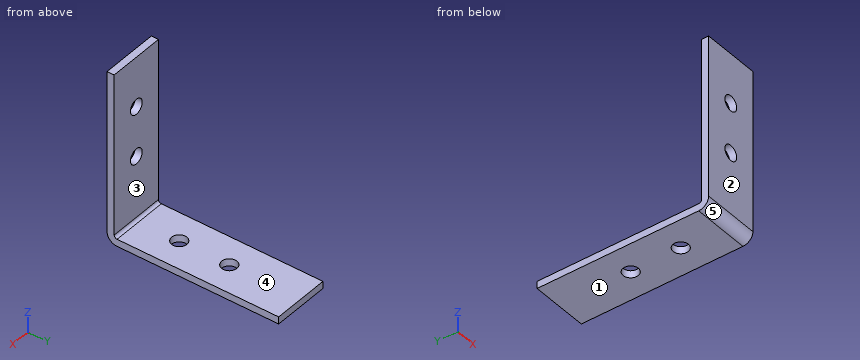
Autodesk Inventor part; units mm, degrees
ref_plane "YZ Plane" through (0, 0, 0) normal (1, 0, 0) x (0, 1, 0)
ref_plane "XZ Plane" through (0, 0, 0) normal (0, 1, 0) x (-1, 0, 0)
ref_plane "XY Plane" through (0, 0, 0) normal (0, 0, 1) x (1, 0, 0)
sketch "Sketch1" plane through (0, 0, 0) normal (0, 0, 1) x (1, 0, 0)
  line L0 (0, 0) -> (147.699314, 0)
  line L1 (147.699314, -25.4) -> (0, -25.4)
  line L2 (0, 0) -> (73.849657, 0)
  line L3 (73.849657, 0) -> (73.849657, -3.175)
  line L4 (73.849657, -3.175) -> (72.249457, -3.175)
  line L5 (72.249457, -3.175) -> (72.249457, -9.525)
  line L6 (72.249457, -9.525) -> (75.424457, -9.525)
  line L7 (75.424457, -9.525) -> (75.424457, -3.175)
  line L8 (75.424457, -3.175) -> (73.849657, -3.175)
  line L9 (73.849657, -25.4) -> (73.849657, -22.225)
  line L10 (73.849657, -22.225) -> (72.249457, -22.225)
  line L11 (72.249457, -22.225) -> (72.249457, -15.875)
  line L12 (72.249457, -15.875) -> (75.424457, -15.875)
  line L13 (75.424457, -15.875) -> (75.424457, -22.225)
  line L14 (75.424457, -22.225) -> (73.849657, -22.225)
  dimension "d8" = 6.7564
sketch "Sketch3" plane through (0, 3.175, 76.2) normal (0, 1, 0) x (1, 0, 0)
  line L0 (0, 0) -> (25.4, 0)
  circle A0 centre (12.7, 44.45) radius 3.3782
  circle A1 centre (12.7, 22.225) radius 3.3782
  line L1 (0, 76.2) -> (0, 73.025)
  dimension "d21" = 6.7564
  dimension "d22" = 6.7564
  dimension "d23" = 12.7
  dimension "d24" = 22.225
  dimension "d25" = 22.225
sketch "Sketch1 outline for Plate1" plane through (0, 0, 0) normal (0, 0, 1) x (1, 0, 0)
  line L0 (0, 0) -> (0, 76.2)
  line L1 (25.4, 0) -> (0, 0)
  line L2 (0, 76.2) -> (25.4, 76.2)
  line L3 (25.4, 76.2) -> (25.4, 0)
  circle A0 centre (12.7, 22.225) radius 3.3782
  circle A1 centre (12.7, 44.45) radius 3.3782
extrude "Plate1" add sketch "Sketch1 outline for Plate1" along normal blind 3.175
sketch "Sketch2" plane through (25.4, 3.175, 0) normal (0, -1, 0) x (1, 0, 0)
  line L0 (-25.4, 0) -> (0, 0)
  line L1 (0, 0) -> (0, 76.2)
  line L2 (0, 76.2) -> (-25.4, 76.2)
  line L3 (-25.4, 76.2) -> (-25.4, 0)
edge flange "Flange1" height 76.2 angle 90 thickness 3.175 bend radius 1.27 thickness toward (0, -1, 0) relief tear relief width 3.175 relief depth 1.5875 edges at (12.7, 0, 3.175) wall of the first edge with corners at (0, 3.175, 0) (25.4, 3.175, 0) (25.4, 3.175, 76.2) (0, 3.175, 76.2)
bend "Bend1"
corner "Corner1"
extrude "Cut1" cut sketch "Sketch3" against normal blind 3.175
equation "\"d11\" = BendReliefWidth"
equation "\"d12\" = BendReliefDepth"
equation "\"d13\" = MinimumRemnant"
equation "\"d14\" = BendRadius"
equation "\"d18\" = CornerReliefSize"
equation "\"d19\" = GapSize"
equation "\"d20\" = JacobiRadiusSize"
equation "\"BendRadius\" = Thickness"
equation "\"BendReliefWidth\" = Thickness"
equation "\"BendReliefDepth\" = 0.5 * Thickness"
equation "\"CornerReliefSize\" = 4 * Thickness"
equation "\"MinimumRemnant\" = 2 * Thickness"
equation "\"TransitionRadius\" = BendRadius"
equation "\"JacobiRadiusSize\" = BendRadius"
equation "\"GapSize\" = Thickness"
equation "\"d10\" = BendRadius"
equation "\"d6\" = Thickness"
properties part number "Rebuild Gusset 4" material "Aluminum 6061"
Work out the finished part from the listing and answer in its coordinate system (mm). Face numbers are marked on the shaded views. A direction names the side the tool comes from. Give positions to 0.01 mm unless a question says otherwise; leave off trailing zeros. Loops run counter-clockwise (first coordinate to the right, second up) from the corner with the lowest first, then second, coordinate; pieces in that order, holes last. Notation, with made-up numbers: (-26, 40.25) -> (8, 40.25) arc R21 ccw to (8, 60.25) -> close; hole circle Ø7 at (23.25, -5.5). An arc over 180 degrees is marked (long way). Use a Markdown table: item, result. Add a question column.
1) Each of these flat-tipped pins is pushed along its axis until it touches: P1, Ø2, axis at x = 5, z = 15, coming from the +Y side (3 decimals); P2, Ø4, axis at x = 22, y = 33, coming from the +Z side (3 decimals). Where does it stop, or does it pass through?
2) The part is cut by section A-A, the plane x = 12.7. Determine the outline of the cut face in (y, z) (3 decimals), plus the area to 3 significant figures.
3) The part is cut by section B-B, the plane z = 31.75. Determine the outline of the cut face in (x, y) (3 decimals), plus the area to 3 significant figures.
4) Consider line 1 along Z through (x, y) = (12.7, 2); line 2 along Y through (x, z) = (12.7, 1.2); line 3 along Y through (x, z) = (5.25, 6) (3 decimals). Determine where each line is inside the solid, lowest interval first.
5) The part is cut by section D-D, the plane y = 42. Determine the outline of the cut face in (x, z) (3 decimals).
6) Which of the six approach directions +Z, -Z, +X, -X, +Y, -Y give full straight-line access (tool end or side, diameter ignored) to the marked faces 4 and 5?
7) For a pull along Y with two mould halves and no side action, classify the marked faces 1, 2 and 3 as +Y half, -Y half, draft (parallel to the pull), parting line (faces both ways), or undercut.
8) The part is cut by section C-C, the plane x = 1.75. Determine the outline of the cut face in (y, z) (3 decimals).
Reported:
| question | item | result |
|---|---|---|
| 1 | P1 | stops at y = 3.175 |
| 1 | P2 | stops at z = 3.175 |
| 2 | outline | (0, 4.445) arc R4.445 ccw to (4.445, 0) -> (18.847, 0) -> (18.847, 3.175) -> (4.445, 3.175) arc R1.27 cw to (3.175, 4.445) -> (3.175, 28.372) -> (0, 28.372) -> close; (0, 35.128) -> (3.175, 35.128) -> (3.175, 50.597) -> (0, 50.597) -> close; (0, 57.353) -> (3.175, 57.353) -> (3.175, 76.2) -> (0, 76.2) -> close; (25.603, 0) -> (41.072, 0) -> (41.072, 3.175) -> (25.603, 3.175) -> close; (47.828, 0) -> (76.2, 0) -> (76.2, 3.175) -> (47.828, 3.175) -> close |
| 2 | area | 384 mm^2 |
| 3 | outline | (0, 0) -> (9.322, 0) -> (9.322, 3.175) -> (0, 3.175) -> close; (16.078, 0) -> (25.4, 0) -> (25.4, 3.175) -> (16.078, 3.175) -> close |
| 3 | area | 59.2 mm^2 |
| 4 | line 1 | z = 0.73 to 28.37, 35.13 to 50.6, 57.35 to 76.2 |
| 4 | line 2 | y = 1.41 to 18.85, 25.6 to 41.07, 47.83 to 76.2 |
| 4 | line 3 | y = 0 to 3.175 |
| 5 | outline | (0, 0) -> (10.374, 0) -> (10.374, 3.175) -> (0, 3.175) -> close; (15.026, 0) -> (25.4, 0) -> (25.4, 3.175) -> (15.026, 3.175) -> close |
| 6 | face 4 | +Z, +X, -X, +Y |
| 6 | face 5 | -Z, +X, -X, -Y |
| 7 | face 1 | draft |
| 7 | face 2 | -Y half |
| 7 | face 3 | +Y half |
| 8 | outline | (0, 4.445) arc R4.445 ccw to (4.445, 0) -> (76.2, 0) -> (76.2, 3.175) -> (4.445, 3.175) arc R1.27 cw to (3.175, 4.445) -> (3.175, 76.2) -> (0, 76.2) -> close |
